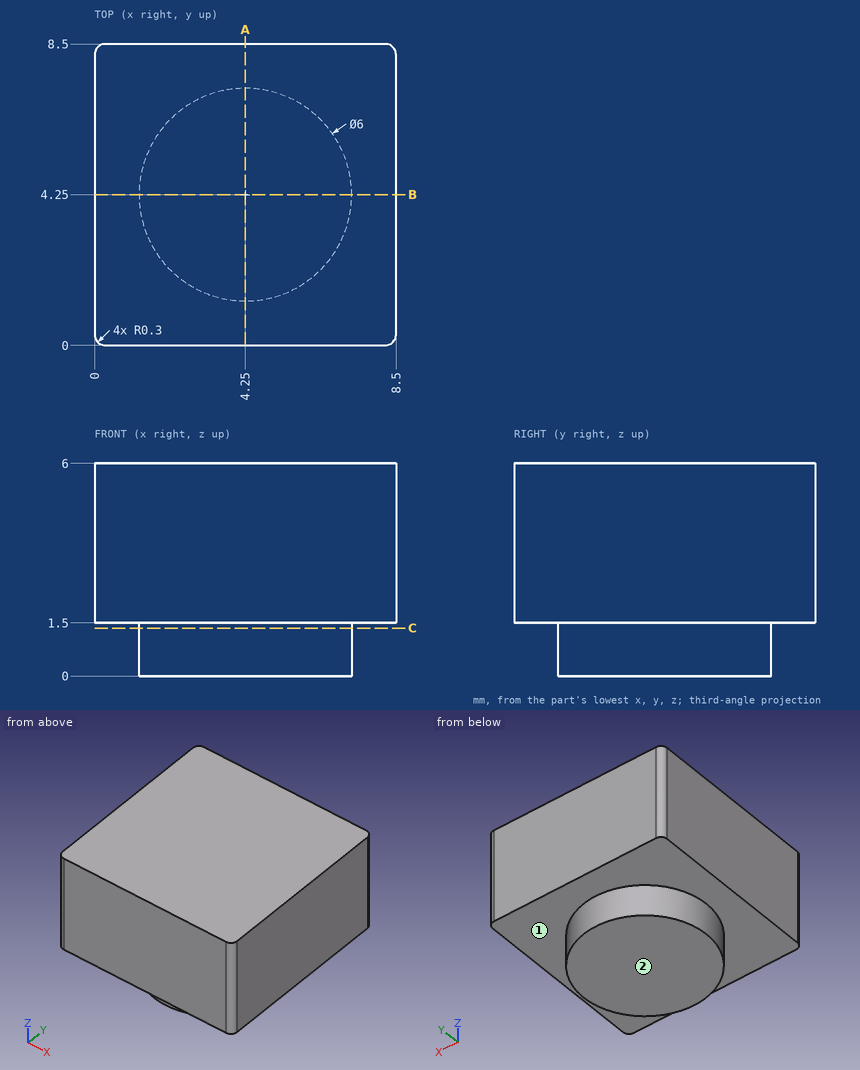
The drawing under review shows one solid part. Ordinate dimensions are in mm from its lowest x, y, z. A direction names the side the tool comes from. Coordinates: 2 decimals unless noted, no trailing zeros. Order: outer loops, then holes, each group sorted by start corner. A loop starts at its lowest first (then second) coordinate and runs counter-clockwise, first axis right, second up. Notation, with made-up numbers: (36.5, 63) -> (63.5, 63) arc R28 ccw to (63.5, 101) -> close; hole circle Ø8 at (-33.75, 26). An arc over 180 degrees is marked (long way). Answer in a Markdown table with one row per item.
(1) Consider section A-A (x = 4.25). Write out the cut boundary in (y, z), plus the area to 4 significant figures.
Answers:
| item | result |
|---|---|
| outline | (0, 1.5) -> (1.25, 1.5) -> (1.25, 0) -> (7.25, 0) -> (7.25, 1.5) -> (8.5, 1.5) -> (8.5, 6) -> (0, 6) -> close |
| area | 47.25 mm² |
(2) Wall thickness on line 1 along Z through (x, y) = (2.25, 0.75); line 2 along Y through (x, z) = (2.75, 1.1); line 3 along Y through (x, z) = (5, 0.9): over which ranges is each line inside the solid? List them lowest first.
Answers:
| item | result |
|---|---|
| line 1 | 1.5 to 6 |
| line 2 | 1.65 to 6.85 |
| line 3 | 1.35 to 7.15 |
(3) Insertion check: pin 1 (1.5 mm diameter, centred on y = 4, z = 4, fed in from -X). The pin has a flat end and moves straight along its axis. Give the tip position at first contact, or say it passes through.
Answers:
| item | result |
|---|---|
| pin 1 | x = 0 |
(4) Consider section C-C (z = 1.35). Write out the cut boundary in (x, y).
Answers:
| item | result |
|---|---|
| outline | circle Ø6 at (4.25, 4.25) |
(5) Machinability: for the marked faces 1 and 2, which of the approach directions +Z, -Z, +X, -X, +Y, -Y give a long, thin tool a straight path to every point of the face, cutting with its end or side? Answer none if there is none.
Answers:
| item | result |
|---|---|
| face 1 | -Z |
| face 2 | -Z, +X, -X, +Y, -Y |
